from build123d import *

# Parameters (mm, degrees)
F0_W     = 203.2
F0_H     = 15.875
F1_DEPTH = 3.175


with BuildPart() as f1:
    # F0 (on Top) → F1 (new body)
    with BuildSketch(Plane.XY):
        with Locations((-101.6, 7.9375)):
            Rectangle(F0_W, F0_H)
        with BuildLine():
            ThreePointArc((-190.5, 3.175), (-193.675, 6.35), (-190.5, 9.525))
            Line((-190.5, 9.525), (-12.7, 9.525))
            ThreePointArc((-12.7, 9.525), (-9.525, 6.35), (-12.7, 3.175))
            Line((-12.7, 3.175), (-190.5, 3.175))
        make_face(mode=Mode.SUBTRACT)
    extrude(amount=F1_DEPTH)


solid = f1.part
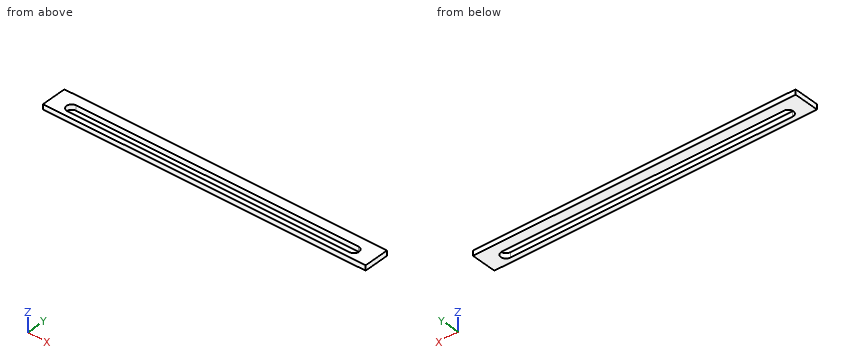
Geometry check sheet. Reference: the model listing, model coordinates, mm. Round coordinates to 2 decimals unless told otherwise and drop trailing zeros. Loops run counter-clockwise (first coordinate to the right, second up) from the corner with the lowest first, then second, coordinate; pieces in that order, holes last.
Item 1: Cross-section at B-B on z = 1.65. Record the boundary of the cut face in (x, y) (3 decimals), then the cut area to 3 significant figures.
Item 2: Thickness scan on line 1 (Y direction, x = -77.5, z = 2.5) (3 decimals); line 2 (X direction, y = 6, z = 1.9); line 3 (X direction, y = 9, z = 2.35). Record the ranges inside material, lowest first.
Item 3: Cross-section at A-A on y = 6.35. Record the boundary of the cut face in (x, z) (3 decimals).
Item 4: Cross-section at C-C on x = -122.5. Record the boundary of the cut face in (y, z) (3 decimals).
Answer sheet:
1. outline: (-203.2, 0) - (0, 0) - (0, 15.875) - (-203.2, 15.875) - close; hole (-190.5, 3.175) - (-12.7, 3.175) arc R3.175 ccw to (-12.7, 9.525) - (-190.5, 9.525) arc R3.175 ccw to start
1. area: 2,070 mm2
2. line 1: y = 0 to 3.175, 9.525 to 15.875
2. line 2: x = -203.2 to -193.66, -9.54 to 0
2. line 3: x = -203.2 to -192.25, -10.95 to 0
3. outline: (-203.2, 0) - (-193.675, 0) - (-193.675, 3.175) - (-203.2, 3.175) - close; (-9.525, 0) - (0, 0) - (0, 3.175) - (-9.525, 3.175) - close
4. outline: (0, 0) - (3.175, 0) - (3.175, 3.175) - (0, 3.175) - close; (9.525, 0) - (15.875, 0) - (15.875, 3.175) - (9.525, 3.175) - close
